Here's how the part is built. I have some questions about the finished solid (model axes, mm). A direction names the side the tool comes from. Give positions to 0.01 mm unless a question says otherwise; leave off trailing zeros. Loops run counter-clockwise (first coordinate to the right, second up) from the corner with the lowest first, then second, coordinate; pieces in that order, holes last.
Q1. I'm going to push flat-ended pins straight in: P1, Ø4, axis at x = 4.5, y = 0, coming from the -Z side; P2, Ø1, axis at x = 2, y = -17, coming from the +Z side; P3, Ø1, axis at x = 1.5, y = 0.5, coming from the +Z side. Where does each tip first touch, or does it pass through?
Q2. Suppose I cut it at C-C (y = -19.5). List the corners of the cut face in (x, z) for me (3 decimals), and give its area (3 significant figures).
Q3. Suppose I cut it at B-B (x = 1.5). List the corners of the cut face in (y, z) for me.
Q4. I need wall thicknesses on probe 1 along Z at (x, y) = (6.5, 0.5); probe 2 along Y at (x, z) = (1.5, -5); probe 3 along Z at (x, y) = (0.5, -12.5). Which ranges of each line are inside material? Lowest first, please.
Q5. Suppose I cut it at A-A (z = 6). List the corners of the cut face in (x, y) for me (3 decimals), and give its area (3 significant figures).
Q6. Thinking about a two-plate mould opening in Z: for faces 1 (the face through (6, 0, -19.732)), 2 (the face through (7, 0, -15.732)), 3 (the face through (0, 0, -26)), 4 (the face through (3, -2.5, -17)), which applies, pulls with the +Z half, pulls with the -Z half, needs draft (parallel to the pull), parting line crosses it, or undercut?
Q7. For faces 5 (the face through (5, 0, -18)), 6 (the face through (2, 31.75, -73)), 7 (the face through (2, 31.75, 22)), which set-ups out of +Z, -Z, +X, -X, +Y, -Y let a thin tool reach every point of the face, with its end or its side?
```python
from build123d import *

# Parameters (mm, degrees)
BOSS_EXTRUDE1_DEPTH = 3.175
BOSS_EXTRUDE2_DEPTH = 5
SKETCH4_W           = 4
SKETCH4_H           = 5
BOSS_EXTRUDE3_DEPTH = 3.175


with BuildPart() as part:
    # Sketch1 → Boss-Extrude1 (new body)
    with BuildSketch(Plane(origin=(0, 0, 0), x_dir=(0, 0, -1), z_dir=(1, 0, 0))):
        Polygon((19.732226513, 31.75), (19.732226513, 0), (32.432226513, 0), (32.432226513, 31.75), (114.982226513, 31.75), (114.982226513, 38.1), (-62.817773487, 38.1), (-62.817773487, 31.75), align=None)
        Polygon((32.432226513, 0), (19.732226513, 0), (19.732226513, -31.75), (-62.817773487, -31.75), (-62.817773487, -38.1), (114.982226513, -38.1), (114.982226513, -31.75), (32.432226513, -31.75), align=None)
    extrude(amount=BOSS_EXTRUDE1_DEPTH)

    # Sketch2 → Boss-Extrude2 (add)
    with BuildSketch(Plane.ZY):
        Polygon((-19.732226513, 5.5), (-19.732226513, 2.5), (-14.732226513, 2.5), (-14.732226513, -2.5), (-19.732226513, -2.5), (-19.732226513, -5.5), (-11.732226513, -5.5), (-11.732226513, 5.5), align=None)
    extrude(amount=-BOSS_EXTRUDE2_DEPTH)

    # Sketch4 → Boss-Extrude3 (add)
    with BuildSketch(Plane(origin=(5, 0, 0), x_dir=(0, 0, -1), z_dir=(1, 0, 0))):
        Polygon((11.732226513, 5.5), (11.732226513, -5.5), (19.732226513, -5.5), (19.732226513, -2.5), (14.732226513, -2.5), (14.732226513, 2.5), (19.732226513, 2.5), (19.732226513, 5.5), align=None)
        with Locations((17.732226513, 0)):
            Rectangle(SKETCH4_W, SKETCH4_H)
    extrude(amount=BOSS_EXTRUDE3_DEPTH)


solid = part.part
```
Solutions:
1. P1: stops at z = -32.43
1. P2: stops at z = -19.73
1. P3: stops at z = -11.73
2. outline: (0, -32.432) - (3.175, -32.432) - (3.175, -19.732) - (0, -19.732) - close
2. area: 40.3 mm2
3. outline: (-38.1, -114.98) - (-31.75, -114.98) - (-31.75, -32.43) - (31.75, -32.43) - (31.75, -114.98) - (38.1, -114.98) - (38.1, 62.82) - (31.75, 62.82) - (31.75, -19.73) - (5.5, -19.73) - (5.5, -11.73) - (-5.5, -11.73) - (-5.5, -19.73) - (-31.75, -19.73) - (-31.75, 62.82) - (-38.1, 62.82) - close; hole (-2.5, -19.73) - (2.5, -19.73) - (2.5, -14.73) - (-2.5, -14.73) - close
4. probe 1: z = -19.73 to -15.73, -14.73 to -11.73
4. probe 2: y = -38.1 to -31.75, 31.75 to 38.1
4. probe 3: z = -32.43 to -19.73
5. outline: (0, -38.1) - (3.175, -38.1) - (3.175, -31.75) - (0, -31.75) - close; (0, 31.75) - (3.175, 31.75) - (3.175, 38.1) - (0, 38.1) - close
5. area: 40.3 mm2
6. face 1: pulls with the -Z half
6. face 2: undercut
6. face 3: needs draft
6. face 4: undercut
7. face 5: -Z, -X
7. face 6: -Z, +X, -X
7. face 7: +Z, +X, -X
